```python
from build123d import *

# Parameters (mm, degrees)
SKETCH1_W           = 130
SKETCH1_H           = 65
SKETCH1_R           = 3
SKETCH1_W_2         = 12
SKETCH1_H_2         = 46
BOSS_EXTRUDE1_DEPTH = 5
FILLET1_R           = 2
SKETCH2_W           = 130
SKETCH2_H           = 5
BOSS_EXTRUDE2_DEPTH = 70
SKETCH3_W           = 5
SKETCH3_H           = 70
BOSS_EXTRUDE3_DEPTH = 60
SKETCH4_R           = 4
SKETCH4_R_2         = 1.5
CUT_EXTRUDE1_DEPTH  = 10
SKETCH5_R           = 8.5
CUT_EXTRUDE2_DEPTH  = 3
SKETCH6_W           = 5
SKETCH6_H           = 70
BOSS_EXTRUDE4_DEPTH = 60
SKETCH7_R           = 19.175
CUT_EXTRUDE3_DEPTH  = 5


with BuildPart() as part:
    # Sketch1 → Boss-Extrude1 (new body)
    with BuildSketch(Plane(origin=(0, 0, 0), x_dir=(1, 0, 0), z_dir=(0, 1, 0))):
        Rectangle(SKETCH1_W, SKETCH1_H)
        with Locations(Location((-45, 20.65, 0), (0, 0, 270))):
            Circle(SKETCH1_R, mode=Mode.SUBTRACT)
        with Locations(Location((-45, -20.65, 0), (0, 0, 90))):
            Circle(SKETCH1_R, mode=Mode.SUBTRACT)
        with Locations(Location((45, 20.65, 0), (0, 0, 90))):
            Circle(SKETCH1_R, mode=Mode.SUBTRACT)
        with Locations(Location((45, -20.65, 0), (0, 0, 270))):
            Circle(SKETCH1_R, mode=Mode.SUBTRACT)
        Rectangle(SKETCH1_W_2, SKETCH1_H_2, mode=Mode.SUBTRACT)
    extrude(amount=BOSS_EXTRUDE1_DEPTH)

    # Fillet1
    fillet1_edges = [part.edges().sort_by_distance(p)[0] for p in [
        (-6, 2.5, -23),
        (-6, 2.5, 23),
        (6, 2.5, 23),
        (6, 2.5, -23),
    ]]
    fillet(fillet1_edges, radius=FILLET1_R)

    # Sketch2 → Boss-Extrude2 (add)
    with BuildSketch(Plane.XZ):
        with Locations((0, -30)):
            Rectangle(SKETCH2_W, SKETCH2_H)
    extrude(amount=BOSS_EXTRUDE2_DEPTH)

    # Sketch3 → Boss-Extrude3 (add)
    with BuildSketch(Plane.XY.offset(-27.5)):
        with Locations((-10, -35)):
            Rectangle(SKETCH3_W, SKETCH3_H)
    extrude(amount=BOSS_EXTRUDE3_DEPTH)

    # Sketch4 → Cut-Extrude1 (cut)
    with BuildSketch(Plane.ZY.offset(12.5)):
        with Locations((0, -35)):
            Circle(SKETCH4_R)
        with Locations((0, -24)):
            Circle(SKETCH4_R_2)
        with Locations((-9.526279442, -29.5)):
            Circle(SKETCH4_R_2)
        with Locations((-9.526279442, -40.5)):
            Circle(SKETCH4_R_2)
        with Locations((0, -46)):
            Circle(SKETCH4_R_2)
        with Locations((9.526279442, -40.5)):
            Circle(SKETCH4_R_2)
        with Locations((9.526279442, -29.5)):
            Circle(SKETCH4_R_2)
    extrude(amount=-CUT_EXTRUDE1_DEPTH, mode=Mode.SUBTRACT)

    # Sketch5 → Cut-Extrude2 (cut)
    with BuildSketch(Plane.ZY.offset(12.5)):
        with Locations((0, -35)):
            Circle(SKETCH5_R)
    extrude(amount=-CUT_EXTRUDE2_DEPTH, mode=Mode.SUBTRACT)

    # Sketch6 → Boss-Extrude4 (add)
    with BuildSketch(Plane.XY.offset(-27.5)):
        with Locations((-62.5, -35)):
            Rectangle(SKETCH6_W, SKETCH6_H)
    extrude(amount=BOSS_EXTRUDE4_DEPTH)

    # Sketch7 → Cut-Extrude3 (cut)
    with BuildSketch(Plane.ZY.offset(65)):
        with Locations((0, -35)):
            Circle(SKETCH7_R)
    extrude(amount=-CUT_EXTRUDE3_DEPTH, mode=Mode.SUBTRACT)


solid = part.part
```
Verification items for the finished model (mm, model axes). A direction names the side the tool comes from. Coordinates: 2 decimals unless noted, no trailing zeros. Write each loop counter-clockwise with the first axis right and the second up, starting at its lowest first coordinate (ties: lowest second). Pieces come first, ordered by that corner, then holes. Notation, with made-up numbers: M 45.5,-22.5 L 66.5,-22.5 A22 cw 66.5,-10.5 Z; hole C 6.25,-15.75 d8. An arc over 180 degrees is marked long. Answer as a JSON object with one key per item and string values. Group by question number.
(1) Material ranges on line 1 (Y direction, x = -10.2, z = 0); line 2 (Y direction, x = -8, z = 0); line 3 (X direction, y = 3.4, z = 20.65), recorded low to high.
(2) Gauge pin test, flat ends, axial feed: pin 1 (3.5 mm diameter, centred on y = -46, z = 0, fed in from -X); pin 2 (1 mm diameter, centred on x = 37, z = -11.5, fed in from -Y); pin 3 (2 mm diameter, centred on y = -40.5, z = -1.5, fed in from +X). Record the tip position at first contact, or that the pin passes through.
(3) Cross-section at A-A, the plane x = 45. Record the cut outline in (y, z).
(4) Cross-section at C-C, the plane y = -63. Record the cut outline in (x, z), and give its area (3 significant figures).
(5) Release check for a two-part mould opening along X. For faces 6 (the face through (-9.5, -37, 4)), 7 (the face through (-15, 5, 0)), 8 (the face through (0, 2, 23)) record: +X half, -X half, draft (parallel to the pull), parting line (faces both ways), or undercut.
(6) Cross-section at B-B, the plane z = 0. State how many separate pieces and enclosed holes the cut face has, and give its area (3 significant figures).
(7) Cross-section at D-D, the plane z = -15. Record the cut outline in (x, y), and give its area (3 significant figures).
(8) Tool access check on faces 1 (the face through (0, 2, -23)), 2 (the face through (-10, -70, -12)), 3 (the face through (-37, 0, 2)), 4 (the face through (-62.54, -15.99, -2.5)), 5 (the face through (28, -35, -27.5)). Record the directions out of +Z, -Z, +X, -X, +Y, -Y that give a thin tool (end or side, any length) a straight path to the whole face; none if there is none.
Reply:
{
 "1": {"line 1": "-70 to -47.5, -44.5 to -43.5, -26.5 to -25.5, -22.5 to 5", "line 2": "-70 to -47.5, -44.5 to -39, -31 to -25.5, -22.5 to 5", "line 3": "-65 to -48, -42 to -6, 6 to 42, 48 to 65"},
 "2": {"pin 1": "x = -12.5", "pin 2": "y = 0", "pin 3": "x = -7.5"},
 "3": {"outline": "M -70,-32.5 L 5,-32.5 L 5,-23.65 L 0,-23.65 L 0,-27.5 L -70,-27.5 Z; M 0,-17.65 L 5,-17.65 L 5,17.65 L 0,17.65 Z; M 0,23.65 L 5,23.65 L 5,32.5 L 0,32.5 Z"},
 "4": {"outline": "M -65,-32.5 L 65,-32.5 L 65,-27.5 L -7.5,-27.5 L -7.5,32.5 L -12.5,32.5 L -12.5,-27.5 L -60,-27.5 L -60,32.5 L -65,32.5 Z", "area": "1,250 mm²"},
 "5": {"face 6": "-X half", "face 7": "draft", "face 8": "undercut"},
 "6": {"separate pieces": "6", "enclosed holes": "0", "area": "1,000 mm²"},
 "7": {"outline": "M -65,-70 L -60,-70 L -60,-46.94 L -65,-46.94 Z; M -65,-23.06 L -60,-23.06 L -60,0 L -12.5,0 L -12.5,-70 L -7.5,-70 L -7.5,0 L -6,0 L -6,5 L -65,5 Z; M 6,0 L 65,0 L 65,5 L 6,5 Z", "area": "1,170 mm²"},
 "8": {"face 1": "+Y, -Y", "face 2": "+Z, -Z, +X, -X, -Y", "face 3": "+Z, -Y", "face 4": "-X", "face 5": "+Z, +X, -Y"}
}
